Autodesk Inventor part; units mm, degrees
ref_plane "YZ Plane" through (0, 0, 0) normal (1, 0, 0) x (0, 1, 0)
ref_plane "XZ Plane" through (0, 0, 0) normal (0, 1, 0) x (-1, 0, 0)
ref_plane "XY Plane" through (0, 0, 0) normal (0, 0, 1) x (1, 0, 0)
sketch "Эскиз1" plane through (0, 0, 0) normal (0, 1, 0) x (-1, 0, 0)
  line L0 (19, -20) -> (-19, -20)
  line L1 (-19, -20) -> (-19, 20)
  line L2 (-19, 20) -> (19, 20) construction
  line L3 (19, 20) -> (19, -20)
  line L4 (37.5, 20) -> (-37.5, 20) construction
  line L5 (-37.5, 20) -> (-37.5, 22)
  line L6 (-37.5, 22) -> (37.5, 22)
  line L7 (37.5, 22) -> (37.5, 20)
  line L8 (19, 20) -> (37.5, 20)
  line L9 (-19, 20) -> (-37.5, 20)
  line L10 (16, -18) -> (-16, -18)
  line L11 (-16, -18) -> (-16, 20)
  line L12 (-16, 20) -> (16, 20)
  line L13 (16, 20) -> (16, -18)
  point P0 (0, 0)
  point P1 (-19, 0)
  point P2 (0, -20)
  point P3 (0, 20)
  point P4 (0, -18)
  dimension "d0" = 38
  dimension "d1" = 40
  dimension "d2" = 75
  dimension "d3" = 2
  dimension "d13" = 3
  dimension "d14" = 2
extrude "Выдавливание1" add sketch "Эскиз1" along normal blind 24
sketch "Эскиз2" plane through (19, 0, 20) normal (1, 0, 0) x (0, 0, -1)
  line L0 (0, 0) -> (0, 24)
  line L1 (40, 0) -> (40, 24)
  line L2 (40, 0) -> (0, 0)
  point P0 (20, 0)
  point P1 (32, 20.5)
  point P2 (32, 3)
  dimension "d15" = 17.5
  dimension "d16" = 32
  dimension "d17" = 3
hole "Отверстие1" at (19, 20.5, -12) at (19, 3, -12) direction (-1, 0, 0) diameter 3.2 end through all
sketch "Эскиз3" plane through (19, 0, 20) normal (1, 0, 0) x (0, 0, -1)
  circle A0 centre (12, 12) radius 12 construction
  line L0 (0, 24) -> (40, 24)
  line L1 (40, 0) -> (0, 0)
  line L2 (0, 0) -> (0, 24)
  circle A1 centre (12, 12) radius 5
  point P0 (20, 0)
  dimension "d18" = 10
extrude "Выдавливание2" cut sketch "Эскиз3" against normal through all
sketch "Эскиз4" plane through (0, 0, 0) normal (0, -1, 0) x (1, 0, 0)
  line L0 (16, -18) -> (-16, -18)
  line L1 (-16, 20) -> (16, 20)
  line L2 (6, -18) -> (-6, -18)
  line L3 (-6, -18) -> (-6, 20)
  line L4 (-6, 20) -> (6, 20)
  line L5 (6, 20) -> (6, -18)
  point P0 (0, 0)
  point P1 (0, -18)
  point P2 (0, 20)
  point P3 (0, -18)
  point P4 (0, 20)
  point P5 (0, -18)
  dimension "d26" = 12
extrude "Выдавливание3" add sketch "Эскиз4" against normal blind 3
sketch "Эскиз5" plane through (6, 0, 20) normal (1, 0, 0) x (0, 0, -1)
  line L0 (0, 0) -> (0, 24)
  line L1 (0, 13) -> (10, 3)
  line L2 (38, 3) -> (0, 3)
  line L3 (40, 24) -> (0, 24)
  line L4 (19, 24) -> (19, 3)
  line L5 (38, 13) -> (28, 3)
  line L6 (38, 13) -> (38, 3)
  line L7 (28, 3) -> (38, 3)
  line L8 (10, 3) -> (0, 3)
  line L9 (0, 3) -> (0, 13)
  point P0 (20, 0)
  dimension "d27" = 45
  dimension "d28" = 10
extrude "Выдавливание4" add sketch "Эскиз5" against normal blind 2 contours L5 L6 L2 | L0 L1 L2
mirror "Зеркальное отражение1" about plane through (0, 0, 0) normal (1, 0, 0) of "Выдавливание4"
sketch "Эскиз6" plane through (0, 3, 0) normal (0, 1, 0) x (1, 0, 0)
  line L0 (-6, 8) -> (-6, -10)
  line L1 (6, -20) -> (6, 18)
  line L2 (-16, 18) -> (-16, -20)
  line L3 (-16, -1) -> (16, -1)
  line L4 (16, 18) -> (16, -20)
  point P0 (0, 0)
  point P1 (0, -16)
  point P2 (0, 14)
  dimension "d38" = 30
hole "Отверстие2" at (0, 3, 16) at (0, 3, -14) direction (0, -1, 0) diameter 3.2 end through all
properties part number "engine_mount"
Design review of the part built by this model. Coordinates are the model's own, in mm. A direction names the side the tool comes from. Coordinates: 2 decimals unless noted, no trailing zeros. Loops run counter-clockwise (first coordinate to the right, second up) from the corner with the lowest first, then second, coordinate; pieces in that order, holes last. Notation, with made-up numbers: (65.25, 21.25) -> (107.25, 21.25) arc R30 ccw to (107.25, 56.25) -> close; hole circle Ø11 at (-3.5, 77). An arc over 180 degrees is marked (long way). Answer as a JSON object with one key per item and string values.
Q1. Take a section at A-A on y = 15. Give the boundary of the cut face in (x, z), plus the area to 3 significant figures.
Answer block:
{"outline": "(-37.5, 20) -> (-19, 20) -> (-19, 12) -> (-16, 12) -> (-16, 20) -> (16, 20) -> (16, 12) -> (19, 12) -> (19, 20) -> (37.5, 20) -> (37.5, 22) -> (-37.5, 22) -> close; (-19, -20) -> (19, -20) -> (19, 4) -> (16, 4) -> (16, -18) -> (-16, -18) -> (-16, 4) -> (-19, 4) -> close", "area": "406 mm^2"}
Q2. Take a section at C-C on x = -7. Give the boundary of the cut face in (y, z).
Answer block:
{"outline": "(0, -20) -> (24, -20) -> (24, -18) -> (0, -18) -> close; (0, 20) -> (24, 20) -> (24, 22) -> (0, 22) -> close"}
Q3. Clearance check with flat-ended pins moving along their axes: pin 1 Ø8 at (y, z) = (6, -11.5) entering from +X; pin 2 Ø9 at (x, y) = (33, 15) entering from -Z; pin 3 Ø8 at (y, z) = (8, -2.5) entering from -X; pin 4 Ø12 at (x, y) = (-21, 20.5) entering from -Z. State where each tip first meets the part, or that it passes through.
Answer block:
{"pin 1": "stops at x = 19", "pin 2": "stops at z = 20", "pin 3": "stops at x = -19", "pin 4": "stops at z = -20"}
Q4. The part is to be moulded in two halves that separate along Z. For faces 6 (the flat face through (0, 12, -20)), 7 (the flat face through (-4, 6, 17)), 8 (the flat face through (-37.5, 12, 21)), say which applies: +Z half, -Z half, draft (parallel to the pull), parting line (faces both ways), or undercut.
Answer block:
{"face 6": "-Z half", "face 7": "undercut", "face 8": "draft"}
Q5. Take a section at B-B on z = 16. Give the boundary of the cut face in (x, y).
Answer block:
{"outline": "(-19, 0) -> (-16, 0) -> (-16, 24) -> (-19, 24) -> close; (-6, 0) -> (-1.6, 0) -> (-1.6, 3) -> (-4, 3) -> (-4, 9) -> (-6, 9) -> close; (1.6, 0) -> (6, 0) -> (6, 9) -> (4, 9) -> (4, 3) -> (1.6, 3) -> close; (16, 0) -> (19, 0) -> (19, 24) -> (16, 24) -> close"}
Q6. Take a section at D-D on z = 7. Give the boundary of the cut face in (x, y).
Answer block:
{"outline": "(-19, 0) -> (-16, 0) -> (-16, 7.1) -> (-19, 7.1) -> close; (-19, 16.9) -> (-16, 16.9) -> (-16, 24) -> (-19, 24) -> close; (-6, 0) -> (6, 0) -> (6, 3) -> (-6, 3) -> close; (16, 0) -> (19, 0) -> (19, 7.1) -> (16, 7.1) -> close; (16, 16.9) -> (19, 16.9) -> (19, 24) -> (16, 24) -> close"}
Q7. Tool access review of faces 1 (the flat face through (6, 2, 1)), 2 (the cylindrical face through (17.48, 2.93, -10.4)), 3 (the flat face through (28, 12, 20)), 4 (the flat face through (0, 12, 20)), 5 (the flat face through (-28, 12, 20)): name each direction out of +Z, -Z, +X, -X, +Y, -Y from which nothing blocks a thin tool from reaching the whole face with its end or side.
Answer block:
{"face 1": "+Y, -Y", "face 2": "+X", "face 3": "-Z, +X, +Y, -Y", "face 4": "+Y", "face 5": "-Z, -X, +Y, -Y"}
Q8. To check wall thickness, follow L1, parallel to X at y = 1.8, z = 16; L2, parallel to Y at x = 17, z = -12; L3, parallel to Z at x = 6.5, y = 1.75. State the ranges of each line that lie inside material, in increasing order.
Answer block:
{"L1": "x = -19 to -16, -6 to -1.6, 1.6 to 6, 16 to 19", "L2": "y = 0 to 1.4, 4.6 to 18.9, 22.1 to 24", "L3": "z = -20 to -18, 20 to 22"}
